```python
from build123d import *

# Parameters (mm, degrees)
SKETCH1_W            = 85
SKETCH1_H            = 70
BOSS_EXTRUDE1_DEPTH  = 2
HOLE1_D              = 22.4
SKETCH5_W            = 28
SKETCH5_H            = 4
BOSS_EXTRUDE2_DEPTH  = 85
BOSS_EXTRUDE3_REACH  = 115.618
SKETCH6_W            = 4
SKETCH6_H            = 28
M4_CLEARANCE_HOLE1_D = 4.8
FILLET1_R            = 2


with BuildPart() as part:
    # Sketch1 → Boss-Extrude1 (new body)
    with BuildSketch(Plane.XY):
        with Locations((42.5, 35)):
            Rectangle(SKETCH1_W, SKETCH1_H)
    extrude(amount=BOSS_EXTRUDE1_DEPTH)

    # Hole1 (through all)
    with Locations(Plane.XY.offset(2)):
        with Locations((42.5, 35)):
            Hole(HOLE1_D / 2)

    # Sketch5 → Boss-Extrude2 (add)
    with BuildSketch(Plane(origin=(85, 0, 0), x_dir=(0, 0, -1), z_dir=(1, 0, 0))):
        with Locations((14, 2)):
            Rectangle(SKETCH5_W, SKETCH5_H)
    extrude(amount=-BOSS_EXTRUDE2_DEPTH)

    # Sketch6 → Boss-Extrude3 (add, up to next)
    with BuildSketch(Plane(origin=(0, 70, 0), x_dir=(1, 0, 0), z_dir=(0, 1, 0)), mode=Mode.PRIVATE) as boss_extrude3_sk1:
        with Locations((83, 14)):
            Rectangle(SKETCH6_W, SKETCH6_H)
    boss_extrude3_tool1 = extrude(boss_extrude3_sk1.sketch, amount=-BOSS_EXTRUDE3_REACH, mode=Mode.PRIVATE) - part.part
    # Sketch6 → Boss-Extrude3 (add, up to next)
    with BuildSketch(Plane(origin=(0, 70, 0), x_dir=(1, 0, 0), z_dir=(0, 1, 0)), mode=Mode.PRIVATE) as boss_extrude3_sk2:
        with Locations((2, 14)):
            Rectangle(SKETCH6_W, SKETCH6_H)
    boss_extrude3_tool2 = extrude(boss_extrude3_sk2.sketch, amount=-BOSS_EXTRUDE3_REACH, mode=Mode.PRIVATE) - part.part
    add(boss_extrude3_tool1.solids().sort_by_distance((83, 70, -14))[0])
    add(boss_extrude3_tool2.solids().sort_by_distance((2, 70, -14))[0])

    # M4 Clearance Hole1 (through all)
    with Locations(Plane(origin=(0, 4, 0), x_dir=(1, 0, 0), z_dir=(0, 1, 0))):
        with Locations((15, 13), (70, 13)):
            Hole(M4_CLEARANCE_HOLE1_D / 2)

    # Fillet1
    fillet1_edges = [part.edges().sort_by_distance(p)[0] for p in [
        (81, 4, -14),
        (81, 37, 0),
        (83, 70, -28),
        (42.5, 4, 0),
        (4, 4, -14),
        (2, 70, -28),
        (4, 37, 0),
        (85, 0, -13),
        (0, 0, -13),
    ]]
    fillet(fillet1_edges, radius=FILLET1_R)


solid = part.part
```
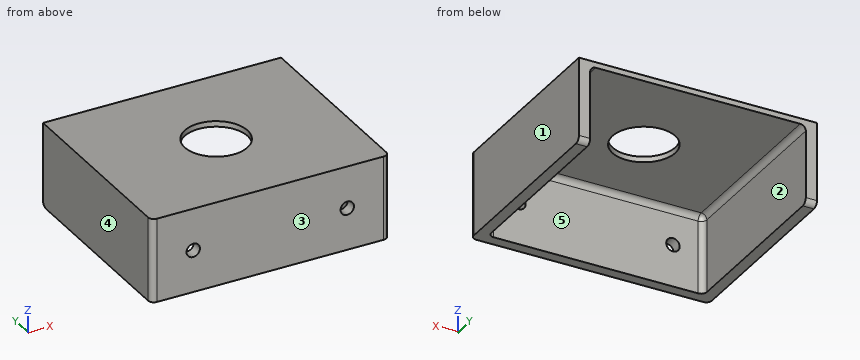
Input: part model. Units: mm. Frame: model coordinates. Face numbers are marked on the shaded views. A direction names the side the tool comes from. Give positions to 0.01 mm unless a question says otherwise; leave off trailing zeros. Write each loop counter-clockwise with the first axis right and the second up, starting at its lowest first coordinate (ties: lowest second). Pieces come first, ordered by that corner, then holes. Notation, with made-up numbers: (3.25, -32.5) - (56.25, -32.5) arc R14 cw to (56.25, -27.5) - close; hole circle Ø4 at (89, 48). An arc over 180 degrees is marked (long way). Write item = value, one per line. Start each with the question number.
1. First-contact query: pin 1 Ø2 at (x, y) = (50.5, 13.5) entering from -Z; pin 2 Ø1 at (x, z) = (24, -16.5) entering from +Y. Flat tips, straight axial feed; report the tip coordinate or a pass-through.
2. Section query C-C, the plane z = -13. Output: boundary loops of the cut face in (x, y).
3. Section query B-B, the plane x = 42.5. Output: boundary loops of the cut face in (y, z), then the cut area to 3 significant figures.
4. Ray query, L1, parallel to Y at x = 42.5, z = 0.9; L2, parallel to X at y = 63, z = -20.25; L3, parallel to Z at x = 15, y = 3.25. Return the intervals inside material, ascending.
5. Section query D-D, the plane z = -17.5. Output: boundary loops of the cut face in (x, y).
6. Access query for the marked faces 4 and 5. Directions: +Z, -Z, +X, -X, +Y, -Y. A direction counts if a zero-diameter tool reaches every point of the face in a straight line with its end or side. Return the directions, or none.
7. Section query A-A, the plane y = 35. Output: boundary loops of the cut face in (x, z), then the cut area to 3 significant figures.
8. Mould query, pull axis X, two halves, no side actions, for the marked faces 1, 2 and 3. Classes: released by +X, released by -X, zero draft, split by the parting line, or undercut.
Check sheet entries:
q1.pin_1 = 0
q1.pin_2 = 4
q2.outline = (0, 2) arc R2 ccw to (2, 0) - (12.6, 0) - (12.6, 4) - (6, 4) arc R2 cw to (4, 6) - (4, 70) - (0, 70) - close; (17.4, 0) - (67.6, 0) - (67.6, 4) - (17.4, 4) - close; (72.4, 0) - (83, 0) arc R2 ccw to (85, 2) - (85, 70) - (81, 70) - (81, 6) arc R2 cw to (79, 4) - (72.4, 4) - close
q3.outline = (0, -28) - (4, -28) - (4, -2) arc R2 cw to (6, 0) - (23.8, 0) - (23.8, 2) - (0, 2) - close; (46.2, 0) - (70, 0) - (70, 2) - (46.2, 2) - close
q3.area = 208 mm2
q4.L1 = 0 to 23.8, 46.2 to 70
q4.L2 = 0 to 4, 81 to 85
q4.L3 = -28 to -15.4, -10.6 to 2
q5.outline = (0, 2) arc R2 ccw to (2, 0) - (83, 0) arc R2 ccw to (85, 2) - (85, 70) - (81, 70) - (81, 6) arc R2 cw to (79, 4) - (6, 4) arc R2 cw to (4, 6) - (4, 70) - (0, 70) - close
q6.face_4 = +Z, -Z, -X, +Y, -Y
q6.face_5 = -Z, +Y
q7.outline = (0, -28) - (4, -28) - (4, -2) arc R2 cw to (6, 0) - (31.3, 0) - (31.3, 2) - (0, 2) - close; (53.7, 0) - (79, 0) arc R2 cw to (81, -2) - (81, -28) - (85, -28) - (85, 2) - (53.7, 2) - close
q7.area = 351 mm2
q8.face_1 = released by +X
q8.face_2 = undercut
q8.face_3 = zero draft
